The model under review builds one solid part; all positions refer to its coordinate system, in mm. Face numbers are marked on the shaded views. A direction names the side the tool comes from. Coordinates: 2 decimals unless noted, no trailing zeros. Loops run counter-clockwise (first coordinate to the right, second up) from the corner with the lowest first, then second, coordinate; pieces in that order, holes last. Notation, with made-up numbers: M 50.25,76.25 L 106.25,76.25 A10 cw 106.25,85.25 Z; hole C -13.5,74 d9. An arc over 180 degrees is marked long. One line per item, written item: value.
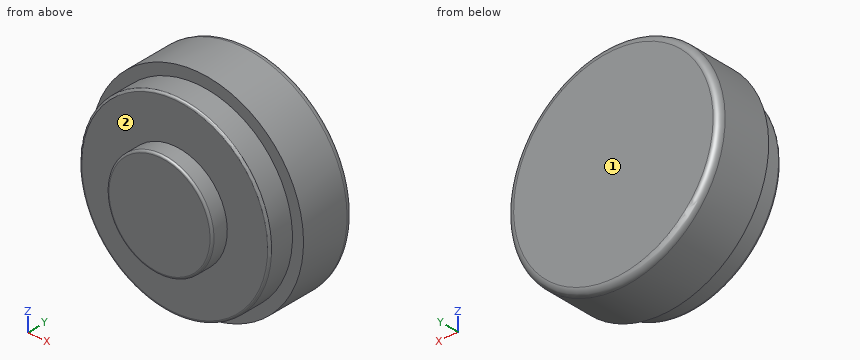
```python
from build123d import *

# Parameters (mm, degrees)
F2_R = 3
F3_R = 1
F4_R = 1


with BuildPart() as f1:
    # F0 (on Right) → F1 (revolve)
    with BuildSketch(Plane.YZ):
        Polygon((-20.8168569952, 49.1500228971), (-20.8168569952, 24.3500228971), (25.1831430048, 24.3500228971), (25.1831430048, 74.3500228971), (-0.8168569952, 74.3500228971), (-0.8168569952, 69.1500228971), (-12.8168569952, 69.1500228971), (-12.8168569952, 49.1500228971), align=None)
    revolve(axis=Axis((0, 2.1831430048, 24.3500228971), (0, 1, 0)))

    # F2
    f2_edges = [f1.edges().sort_by_distance(p)[0] for p in [
        (0, 25.183143, -25.649977),
    ]]
    fillet(f2_edges, radius=F2_R)

    # F3
    f3_edges = [f1.edges().sort_by_distance(p)[0] for p in [
        (0, -12.816857, -20.449977),
    ]]
    fillet(f3_edges, radius=F3_R)

    # F4
    f4_edges = [f1.edges().sort_by_distance(p)[0] for p in [
        (0, -20.816857, -0.449977),
    ]]
    fillet(f4_edges, radius=F4_R)


solid = f1.part
```
(1) Insertion check: pin 1 Ø12 at (x, y) = (26, 3) entering from -Z; pin 2 Ø1 at (y, z) = (-7, 7) entering from -X; pin 3 Ø1.5 at (y, z) = (8.5, 28.5) entering from +X. Each pin has a flat end and moves straight along its axis. Give the tip position at first contact, or say it passes through.
Checks:
pin 1: z = -21.48
pin 2: x = -41.51
pin 3: x = 49.88
(2) Add section A-A on x = 0. State the section outline as (y, z) points.
Checks:
outline: M -20.82,0.55 A1 ccw -19.82,-0.45 L -12.82,-0.45 L -12.82,-19.45 A1 ccw -11.82,-20.45 L -0.82,-20.45 L -0.82,-25.65 L 22.18,-25.65 A3 ccw 25.18,-22.65 L 25.18,71.35 A3 ccw 22.18,74.35 L -0.82,74.35 L -0.82,69.15 L -11.82,69.15 A1 ccw -12.82,68.15 L -12.82,49.15 L -19.82,49.15 A1 ccw -20.82,48.15 Z
(3) Add section C-C on y = -4. State the section outline as (x, z) points.
Checks:
outline: C 0,24.35 d89.6
(4) To check wall thickness, follow L1, parallel to Y at x = -30, z = 17.5; L2, parallel to Y at x = -36.5, z = 54; L3, parallel to X at y = -1, z = 39. State the ranges of each line that lie inside material, in increasing order. Write a range as [from, to].
Checks:
L1: [-12.82, 25.18]
L2: [-0.82, 25.18]
L3: [-42.34, 42.34]
(5) Tool access review of the marked faces 1 and 2: name each direction out of +Z, -Z, +X, -X, +Y, -Y from which nothing blocks a thin tool from reaching the whole face with its end or side.
Checks:
face 1: +Z, -Z, +X, -X, +Y
face 2: -Y
(6) Add section B-B on y = 16. State the section outline as (x, z) points, then the cut area to 3 significant figures.
Checks:
outline: C 0,24.35 d100
area: 7,850 mm^2
